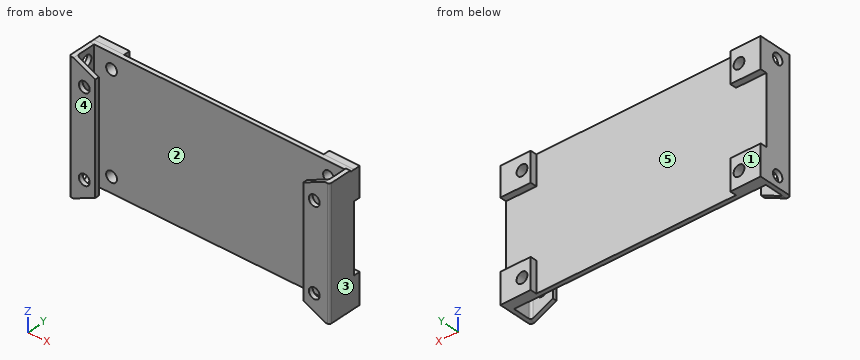
```python
from build123d import *

# Parameters (mm, degrees)
BOSS_EXTRUDE1_DEPTH = 2
SKETCH2_W           = 59.326153163
SKETCH2_H           = 11
BOSS_EXTRUDE2_DEPTH = 2
FILLET1_R           = 1
SKETCH3_R           = 2.5
BOSS_EXTRUDE3_DEPTH = 2
FILLET3_R           = 1
SKETCH4_R           = 2.5
CUT_EXTRUDE1_DEPTH  = 2
BOSS_EXTRUDE5_START = 2
SKETCH3_5_W         = 14
SKETCH3_5_H         = 14
SKETCH3_5_R         = 2.5
BOSS_EXTRUDE5_DEPTH = 3
SKETCH5_R           = 2.5
CUT_EXTRUDE2_DEPTH  = 2


with BuildPart() as part:
    # Sketch1 → Boss-Extrude1 (new body)
    with BuildSketch(Plane(origin=(0, 0, 0), x_dir=(1, 0, 0), z_dir=(0, 1, 0))):
        Polygon((-49.061898328, -3.336557388), (-49.061898328, -53.336557388), (-59.061898328, -57.999633969), (-59.061898328, 1.326519194), align=None)
    boss_extrude1 = extrude(amount=BOSS_EXTRUDE1_DEPTH)

    # Sketch2 → Boss-Extrude2 (add)
    with BuildSketch(Plane.ZY.offset(59.061898328)):
        with Locations((28.336557388, 5.5)):
            Rectangle(SKETCH2_W, SKETCH2_H)
    boss_extrude2 = extrude(amount=BOSS_EXTRUDE2_DEPTH)

    # Fillet1
    fillet1_edges = [part.edges().sort_by_distance(p)[0] for p in [
        (-61.061898328, 0, 28.336557388),
        (-59.061898328, 2, 28.336557388),
    ]]
    fillet(fillet1_edges, radius=FILLET1_R)

    # Sketch3 → Boss-Extrude3 (add)
    with BuildSketch(Plane(origin=(0, 11, 0), x_dir=(1, 0, 0), z_dir=(0, 1, 0))):
        Polygon((-61.061898328, 1.326519194), (-61.061898328, -57.999633969), (58.938101672, -57.413440129), (58.938101672, 1.326519194), align=None)
        with Locations(Location((-51.061898328, -5.673480806, 0), (0, 0, 270))):
            Circle(SKETCH3_R, mode=Mode.SUBTRACT)
        with Locations(Location((48.938101672, -5.673480806, 0), (0, 0, 270))):
            Circle(SKETCH3_R, mode=Mode.SUBTRACT)
        with Locations(Location((-51.061898328, -50.999633969, 0), (0, 0, 270))):
            Circle(SKETCH3_R, mode=Mode.SUBTRACT)
        with Locations(Location((48.938101672, -50.999633969, 0), (0, 0, 270))):
            Circle(SKETCH3_R, mode=Mode.SUBTRACT)
    extrude(amount=BOSS_EXTRUDE3_DEPTH)

    # Mirror1: Boss-Extrude2 across plane
    add(boss_extrude2.mirror(Plane.ZY.offset(1.061898328)))

    # Mirror2: Boss-Extrude1 across plane
    add(boss_extrude1.mirror(Plane.ZY.offset(1.061898328)))

    # Fillet3
    fillet3_edges = [part.edges().sort_by_distance(p)[0] for p in [
        (58.938101672, 0, 28.336557388),
        (56.938101672, 2, 28.336557388),
    ]]
    fillet(fillet3_edges, radius=FILLET3_R)

    # Sketch4 → Cut-Extrude1 (cut)
    with BuildSketch(Plane.ZY.offset(61.061898328)):
        with Locations((3.673480806, 7)):
            Circle(SKETCH4_R)
        with Locations(Location((52.999633969, 7, 0), (0, 0, 180))):
            Circle(SKETCH4_R)
    extrude(amount=-CUT_EXTRUDE1_DEPTH, mode=Mode.SUBTRACT)

    # Sketch3<5> → Boss-Extrude5 (add)
    # profile 1 of 4: a face of its own
    with BuildSketch(Plane(origin=(0, 11, 0), x_dir=(1, 0, 0), z_dir=(0, 1, 0)).offset(BOSS_EXTRUDE5_START)):
        with Locations((-54.061898328, -5.673480806)):
            Rectangle(SKETCH3_5_W, SKETCH3_5_H)
        with Locations(Location((-51.061898328, -5.673480806, 0), (0, 0, 270))):
            Circle(SKETCH3_5_R, mode=Mode.SUBTRACT)
    # profile 2 of 4: a face of its own
    with BuildSketch(Plane(origin=(0, 11, 0), x_dir=(1, 0, 0), z_dir=(0, 1, 0)).offset(BOSS_EXTRUDE5_START)):
        with Locations((51.938101672, -5.673480806)):
            Rectangle(SKETCH3_5_W, SKETCH3_5_H)
        with Locations(Location((48.938101672, -5.673480806, 0), (0, 0, 270))):
            Circle(SKETCH3_5_R, mode=Mode.SUBTRACT)
    # profile 3 of 4: a face of its own
    with BuildSketch(Plane(origin=(0, 11, 0), x_dir=(1, 0, 0), z_dir=(0, 1, 0)).offset(BOSS_EXTRUDE5_START)):
        Polygon((-47.061898328, -43.999633969), (-61.061898328, -43.999633969), (-61.061898328, -57.999633969), (-47.061898328, -57.931244688), align=None)
        with Locations(Location((-51.061898328, -50.999633969, 0), (0, 0, 270))):
            Circle(SKETCH3_5_R, mode=Mode.SUBTRACT)
    # profile 4 of 4: a face of its own
    with BuildSketch(Plane(origin=(0, 11, 0), x_dir=(1, 0, 0), z_dir=(0, 1, 0)).offset(BOSS_EXTRUDE5_START)):
        Polygon((58.938101672, -57.413440129), (58.938101672, -43.999633969), (44.938101672, -43.999633969), (44.938101672, -57.481829411), align=None)
        with Locations(Location((48.938101672, -50.999633969, 0), (0, 0, 270))):
            Circle(SKETCH3_5_R, mode=Mode.SUBTRACT)
    extrude(amount=BOSS_EXTRUDE5_DEPTH)

    # Sketch5 → Cut-Extrude2 (cut)
    with BuildSketch(Plane.XZ):
        with Locations(Location((-54.061898328, 47.903918034, 0), (0, 0, 270))):
            Circle(SKETCH5_R)
        with Locations(Location((51.938101672, 47.903918034, 0), (0, 0, 270))):
            Circle(SKETCH5_R)
        with Locations(Location((51.938101672, 8.769196741, 0), (0, 0, 270))):
            Circle(SKETCH5_R)
        with Locations(Location((-54.061898328, 8.769196741, 0), (0, 0, 270))):
            Circle(SKETCH5_R)
    extrude(amount=-CUT_EXTRUDE2_DEPTH, mode=Mode.SUBTRACT)


solid = part.part
```
CAD build for the part. Positions are in the model's coordinates, mm. Face numbers are marked on the shaded views. A direction names the side the tool comes from. Round coordinates to 2 decimals unless told otherwise and drop trailing zeros. Order: outer loops, then holes, each group sorted by start corner. A loop starts at its lowest first (then second) coordinate and runs counter-clockwise, first axis right, second up.
Q1. Which spindle directions (+Z, -Z, +X, -X, +Y, -Y) get a long thin tool onto all of the face, cutting with end or side? Do the marked faces 1 and 2. Say none if no direction does.
Q2. Slice it at A-A (y = 7). Write the cut outline in (x, z).
Q3. Slice it at C-C (x = 10.5). Write the cut outline in (y, z), and give its area (3 significant figures).
Q4. Two-plate mould, pull along X, no slides. Class the marked faces 3, 4 and 5: pulls with the +X half, pulls with the -X half, needs draft (parallel to the pull), parting line crosses it, or undercut.
Q5. Wall check: L1, parallel to X at y = 10.5, z = 31; L2, parallel to Y at x = -55, z = 40; L3, parallel to X at y = 15, z = 52.5. Give the ranges that are in metal, low to high.
Q6. Drop flat-ended pins along their axis: pin 1 (8 mm diameter, centred on x = -26.5, z = 23, fed in from -Y); pin 2 (4.5 mm diameter, centred on x = -51.06, z = 51, fed in from +Y); pin 3 (8 mm diameter, centred on x = 18.5, z = 24, fed in from +Y). Give the stop position or say it passes through.
Q7. Slice it at B-B (z = 33). Write the cut outline in (x, y).
Q8. Slice it at D-D (x = -14). Write the cut outline in (y, z).
Results below:
1. face 1: +Z, -Z, +X, -X, +Y
1. face 2: +Z, -Z
2. outline: (-61.06, -1.33) - (-59.06, -1.33) - (-59.06, 1.17) - (-61.06, 1.17) - close; (-61.06, 6.17) - (-59.06, 6.17) - (-59.06, 50.5) - (-61.06, 50.5) - close; (-61.06, 55.5) - (-59.06, 55.5) - (-59.06, 58) - (-61.06, 58) - close; (56.94, -1.33) - (58.94, -1.33) - (58.94, 58) - (56.94, 58) - close
3. outline: (11, -1.33) - (13, -1.33) - (13, 57.65) - (11, 57.65) - close
3. area: 118 mm2
4. face 3: pulls with the +X half
4. face 4: needs draft
4. face 5: undercut
5. L1: x = -61.06 to -59.06, 56.94 to 58.94
5. L2: y = 0 to 2, 11 to 13
5. L3: x = -61.06 to -53.06, -49.06 to -47.06, 44.94 to 46.94, 50.94 to 58.94
6. pin 1: stops at y = 11
6. pin 2: stops at y = 2
6. pin 3: stops at y = 13
7. outline: (-61.06, 1) arc R1 ccw to (-60.06, 0) - (-49.06, 0) - (-49.06, 2) - (-58.06, 2) arc R1 cw to (-59.06, 3) - (-59.06, 11) - (56.94, 11) - (56.94, 3) arc R1 cw to (55.94, 2) - (46.94, 2) - (46.94, 0) - (57.94, 0) arc R1 ccw to (58.94, 1) - (58.94, 13) - (-61.06, 13) - close
8. outline: (11, -1.33) - (13, -1.33) - (13, 57.77) - (11, 57.77) - close
